from build123d import *

# Parameters (mm, degrees)
F0_W      = 120
F0_H      = 120
F1_DEPTH  = 50
F2_SIZE   = 35
F4_DEPTH  = 12.5
F6_DEPTH  = 12.5
F7_R      = 15
F8_DEPTH  = 37.501
F9_R      = 14.1
F10_DEPTH = 50.001
F11_SIZE  = 5


with BuildPart() as f1:
    # F0 (on Top) → F1 (new body)
    with BuildSketch(Plane.XY):
        with Locations((3.824193, -6.655599)):
            Rectangle(F0_W, F0_H)
    extrude(amount=F1_DEPTH)

    # F2
    f2_edges = [f1.edges().sort_by_distance(p)[0] for p in [
        (-56.175807, -66.655599, 25),
        (63.824193, -66.655599, 25),
    ]]
    chamfer(f2_edges, length=F2_SIZE)

    # F3 (on face) → F4 (cut)
    with BuildSketch(Plane.XY.offset(50)):
        Polygon((63.824193, -31.655599), (-56.175807, -31.655599), (-21.175807, -66.655599), (28.824193, -66.655599), align=None)
    extrude(amount=-F4_DEPTH, mode=Mode.SUBTRACT)

    # F5 (on face) → F6 (cut)
    with BuildSketch(Plane(origin=(0, 0, 0), x_dir=(1, 0, 0), z_dir=(0, 0, -1))):
        Polygon((-56.175807, 31.655599), (63.824193, 31.655599), (28.824193, 66.655599), (-21.175807, 66.655599), align=None)
    extrude(amount=-F6_DEPTH, mode=Mode.SUBTRACT)

    # F7 (on face) → F8 (cut, through all)
    with BuildSketch(Plane.XY.offset(37.5)):
        with Locations((3.824193, -49.155599)):
            Circle(F7_R)
    extrude(amount=-F8_DEPTH, mode=Mode.SUBTRACT)

    # F9 (on face) → F10 (cut, through all)
    with BuildSketch(Plane.XY.offset(50)):
        with Locations((-25.175807, 23.344401)):
            Circle(F9_R)
        with Locations((32.824193, 23.344401)):
            Circle(F9_R)
    extrude(amount=-F10_DEPTH, mode=Mode.SUBTRACT)

    # F11
    f11_edges = [f1.edges().sort_by_distance(p)[0] for p in [
        (63.824193, 53.344401, 25),
        (-56.175807, 53.344401, 25),
    ]]
    chamfer(f11_edges, length=F11_SIZE)


solid = f1.part
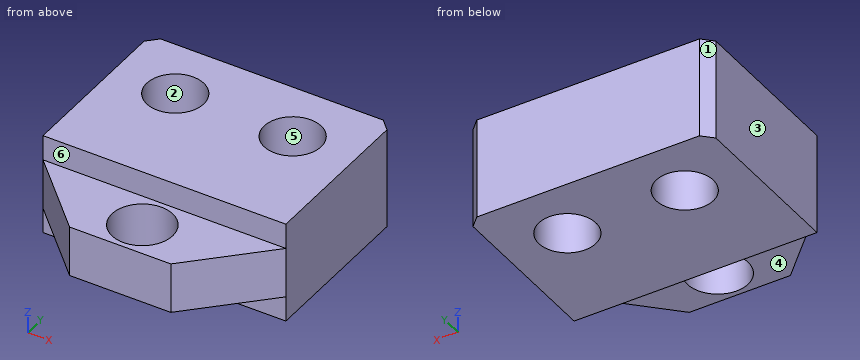
Check sheet for the modelled part. Datum: model origin and axes. Units: mm. Face numbers are marked on the shaded views. A direction names the side the tool comes from. Give positions to 0.01 mm unless a question says otherwise; leave off trailing zeros. Write each loop counter-clockwise with the first axis right and the second up, starting at its lowest first coordinate (ties: lowest second). Pieces come first, ordered by that corner, then holes. Notation, with made-up numbers: (38.25, 52) -> (79.25, 52) arc R19 cw to (79.25, 78) -> close; hole circle Ø11 at (15.25, 88.25). An arc over 180 degrees is marked (long way). Write item = value, one per line.
Item 1: Gauge pin test, flat ends, axial feed: pin 1 (22.5 mm diameter, centred on x = 32.82, y = 23.34, fed in from +Z); pin 2 (6 mm diameter, centred on x = -9, z = 43, fed in from -Y); pin 3 (3 mm diameter, centred on x = -25.5, y = -38, fed in from +Z). Record the tip position at first contact, or that the pin passes through.
Output:
pin_1 = through
pin_2 = -31.66
pin_3 = 37.5
Item 2: Scan lines: probe 1 along Y at (x, z) = (-2.5, 45); probe 2 along Z at (x, y) = (53.5, -39); probe 3 along Y at (x, z) = (-23, 13). Record each from-to range of solid material in increasing order. Write a range as from..to.
Output:
probe_1 = -31.66..53.34
probe_2 = 12.5..37.5
probe_3 = -64.83..9.41, 37.28..53.34
Item 3: Sectioned sample at B-B on y = 19.5. Record the boundary of the cut face in (x, z), and give its area (3 significant figures).
Output:
outline = (-56.18, 0) -> (-38.74, 0) -> (-38.74, 50) -> (-56.18, 50) -> close; (-11.61, 0) -> (19.26, 0) -> (19.26, 50) -> (-11.61, 50) -> close; (46.39, 0) -> (63.82, 0) -> (63.82, 50) -> (46.39, 50) -> close
area = 3,290 mm^2
Item 4: Sectioned sample at D-D on x = 53. Record the boundary of the cut face in (y, z).
Output:
outline = (-42.48, 12.5) -> (-31.66, 12.5) -> (-31.66, 0) -> (53.34, 0) -> (53.34, 50) -> (-31.66, 50) -> (-31.66, 37.5) -> (-42.48, 37.5) -> close
Item 5: Release check for a two-part mould opening along Y. For the marked faces 1, 2 and 3 record: +Y half, -Y half, draft (parallel to the pull), parting line (faces both ways), or undercut.
Output:
face_1 = +Y half
face_2 = undercut
face_3 = draft
Item 6: Tool access check on the marked faces 4, 5 and 6. Record the directions out of +Z, -Z, +X, -X, +Y, -Y that give a thin tool (end or side, any length) a straight path to the whole face; none if there is none.
Output:
face_4 = -Z, +X, -X, -Y
face_5 = +Z, -Z
face_6 = +Z, +X, -X, -Y
Item 7: Sectioned sample at A-A on x = 5. Record the boundary of the cut face in (y, z).
Output:
outline = (-66.66, 12.5) -> (-64.11, 12.5) -> (-64.11, 37.5) -> (-66.66, 37.5) -> close; (-34.2, 12.5) -> (-31.66, 12.5) -> (-31.66, 0) -> (53.34, 0) -> (53.34, 50) -> (-31.66, 50) -> (-31.66, 37.5) -> (-34.2, 37.5) -> close
Item 8: Sectioned sample at C-C on z = 16. Record the boundary of the cut face in (x, y).
Output:
outline = (-56.18, -31.66) -> (-21.18, -66.66) -> (28.82, -66.66) -> (63.82, -31.66) -> (63.82, 48.34) -> (58.82, 53.34) -> (-51.18, 53.34) -> (-56.18, 48.34) -> close; hole circle Ø28.2 at (-25.18, 23.34); hole circle Ø30 at (3.82, -49.16); hole circle Ø28.2 at (32.82, 23.34)
